Here's how the part is built. I have some questions about the finished solid (model axes, mm). Face numbers are marked on the shaded views. Round coordinates to 2 decimals unless told otherwise and drop trailing zeros. Loops run counter-clockwise (first coordinate to the right, second up) from the corner with the lowest first, then second, coordinate; pieces in that order, holes last. Notation, with made-up numbers: M 39,-1 L 78,-1 A13 ccw 78,11 Z; hole C 56,-3.5 d11. An arc over 180 degrees is marked long. Answer as CSV lines item,"result".
```python
from build123d import *

# Parameters (mm, degrees)
ENL_V_MAT_EXTRU_1_DEPTH = 2


with BuildPart() as part:
    # Esquisse1 → Révolution1 (revolve)
    with BuildSketch(Plane.XY):
        with BuildLine():
            Line((0, 3.8), (-2.9, 3.8))
            ThreePointArc((-2.9, 3.8), (-3.253553391, 3.653553391), (-3.4, 3.3))
            Line((-3.4, 3.3), (-3.4, 0))
            Line((-3.4, 0), (-1.95, 0))
            Line((-1.95, 0), (-1.95, -38.5))
            Line((-1.95, -38.5), (-1.45, -39))
            Line((-1.45, -39), (0, -39))
            Line((0, -39), (0, 3.8))
        make_face()
    revolve(axis=Axis((0, 3.8, 0), (0, -1, 0)))

    # Esquisse2 → Enlèv. mat.-Extru.1 (cut)
    with BuildSketch(Plane(origin=(0, 3.8, 0), x_dir=(-1, 0, 0), z_dir=(0, 1, 0))):
        Polygon((-1.732050808, 0), (-0.866025404, -1.5), (0.866025404, -1.5), (1.732050808, 0), (0.866025404, 1.5), (-0.866025404, 1.5), align=None)
    extrude(amount=-ENL_V_MAT_EXTRU_1_DEPTH, mode=Mode.SUBTRACT)


solid = part.part
```
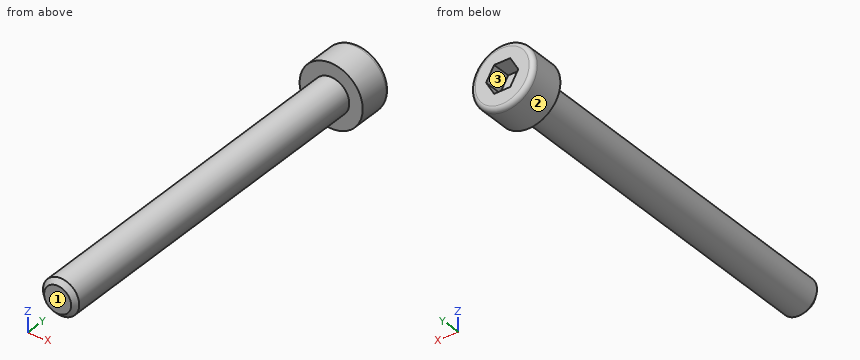
1. We'd pull the mould along X, two halves only. Please class the marked faces 1, 2 and 3: pulls with the +X half, pulls with the -X half, needs draft (parallel to the pull), parting line crosses it, or undercut.
Evaluation:
face 1,"needs draft"
face 2,"parting line crosses it"
face 3,"undercut"
2. If I drill on line 1 (Y direction, x = -0.5, z = 0.75); line 2 (X direction, y = -26.5, z = -1.25); line 3 (Y direction, x = -0.25, z = 2), over which ranges is the centre line in solid material (lowest first)? Write a range as [from, to].
Evaluation:
line 1,"y = [-39, 1.8]"
line 2,"x = [-1.5, 1.5]"
line 3,"y = [0, 3.8]"
3. I want a section at B-B, the plane y = -18.5. Please give me the cut outline in (x, z), and give its area (3 significant figures).
Evaluation:
outline,"C 0,0 d3.9"
area,"11.9 mm²"
4. For P1, Ø1.5, axis at x = 0.5, y = -34.5, coming from the +Z side; P2, Ø4, axis at y = -16.5, z = 0, coming from the +X side; P3, Ø3, axis at x = 2, y = -24.5, coming from the -Z side, each with a flat end and sliding along its axis, tell me the tip position at first contact or that it passes through.
Evaluation:
P1,"stops at z = 1.95"
P2,"stops at x = 1.95"
P3,"stops at z = -1.88"
5. I want a section at A-A, the plane x = 0. Please give me the cut outline in (y, z), and give its area (3 significant figures).
Evaluation:
outline,"M -39,-1.45 L -38.5,-1.95 L 0,-1.95 L 0,-3.4 L 3.3,-3.4 A0.5 ccw 3.8,-2.9 L 3.8,-1.5 L 1.8,-1.5 L 1.8,1.5 L 3.8,1.5 L 3.8,2.9 A0.5 ccw 3.3,3.4 L 0,3.4 L 0,1.95 L -38.5,1.95 L -39,1.45 Z"
area,"172 mm²"
